Source: CAD feature listing. Evaluate the final solid. Frame: model axes, mm. A direction names the side the tool comes from. Give positions to 0.01 mm unless a question says otherwise; leave off trailing zeros. Order: outer loops, then holes, each group sorted by start corner. A loop starts at its lowest first (then second) coordinate and runs counter-clockwise, first axis right, second up.
```python
from build123d import *

# Parameters (mm, degrees)
F0_W     = 47.625
F0_H     = 19.05
F1_DEPTH = 12.7
F3_DEPTH = 7.62
F4_W     = 19.05
F4_H     = 12.7
F5_DEPTH = 7.62
F7_DEPTH = 5.08
F8_R     = 1.27


with BuildPart() as f1:
    # F0 (on Top) → F1 (new body)
    with BuildSketch(Plane.XY):
        Rectangle(F0_W, F0_H)
    extrude(amount=F1_DEPTH)

    # F2 (on face) → F3 (cut)
    with BuildSketch(Plane.XY.offset(12.7)):
        Polygon((-17.4625, -7.62), (-2.2225, -7.62), (-2.2225, 0), (-2.2225, 7.62), (-17.4625, 7.62), align=None)
    extrude(amount=-F3_DEPTH, mode=Mode.SUBTRACT)

    # F4 (on face) → F5 (join)
    with BuildSketch(Plane(origin=(-23.8125, 0, 0), x_dir=(0, -1, 0), z_dir=(-1, 0, 0))):
        with Locations((0, 6.35)):
            Rectangle(F4_W, F4_H)
    extrude(amount=F5_DEPTH)

    # F6 (on face) → F7 (join)
    with BuildSketch(Plane.XY.offset(12.7)):
        Polygon((-28.2575, 3.175), (-31.4325, 3.175), (-31.4325, -3.175), (-25.0825, -3.175), (-25.0825, 3.175), align=None)
    extrude(amount=F7_DEPTH)

    # F8
    f8_edges = [f1.edges().sort_by_distance(p)[0] for p in [
        (-31.4325, 0, 17.78),
        (-25.0825, 0, 17.78),
        (-25.0825, -3.175, 15.24),
        (-28.2575, -3.175, 17.78),
        (-28.2575, 3.175, 17.78),
        (-31.4325, -3.175, 15.24),
        (-28.2575, -3.175, 12.7),
        (-25.0825, 0, 12.7),
        (-28.2575, 3.175, 12.7),
        (-31.4325, 3.175, 15.24),
        (-25.0825, 3.175, 15.24),
        (-31.4325, -6.35, 12.7),
        (-31.4325, 6.35, 12.7),
    ]]
    fillet(f8_edges, radius=F8_R)


solid = f1.part
```
1) Section query A-A, the plane z = 6. Return the cut outline in (x, y) (1 decimal).
Report:
outline: (-31.4, -9.5) - (23.8, -9.5) - (23.8, 9.5) - (-31.4, 9.5) - close; hole (-17.5, -7.6) - (-2.2, -7.6) - (-2.2, 7.6) - (-17.5, 7.6) - close
2) Section query B-B, the plane y = -5.25. Return the cut outline in (x, z), and give its area (3 significant figures).
Report:
outline: (-31.43, 0) - (23.81, 0) - (23.81, 12.7) - (-2.22, 12.7) - (-2.22, 5.08) - (-17.46, 5.08) - (-17.46, 12.7) - (-30.16, 12.7) arc R1.27 ccw to (-31.43, 11.43) - close
area: 585 mm2
3) Reachability of faces 5 (the cylindrical face through (-31.07, -7.02, 12.32)), 6 (the flat face through (-25.082, 0, 15)), 7 (the cylindrical face through (-31.07, 2.793, 15.258)) from +Z, -Z, +X, -X, +Y, -Y: full face, straight path, thin tool, end or side. Return the list, or none.
Report:
face 5: +Z, -X, -Y
face 6: +Z, +X, +Y, -Y
face 7: +Z, -X, +Y
4) Pin query (flat end, axial travel): pin 1 (2 mm diameter, centred on y = -0.5, z = 15.5, fed in from +X); pin 2 (2 mm diameter, centred on x = -29, z = 15, fed in from +Y) (3 decimals); pin 3 (2 mm diameter, centred on x = -27.5, z = 16, fed in from -Y) (3 decimals). Return the tip coordinate at first contact, or that it passes through.
Report:
pin 1: stops at x = -25.08
pin 2: stops at y = 3.175
pin 3: stops at y = -3.175
5) Section query D-D, the plane z = 15. Return the cut outline in (x, y) (1 decimal), and give its area (3 significant figures).
Report:
outline: (-31.4, -1.9) arc R1.3 ccw to (-30.2, -3.2) - (-26.4, -3.2) arc R1.3 ccw to (-25.1, -1.9) - (-25.1, 1.9) arc R1.3 ccw to (-26.4, 3.2) - (-30.2, 3.2) arc R1.3 ccw to (-31.4, 1.9) - close
area: 38.9 mm2
6) Section query C-C, the plane x = -10. Return the cut outline in (y, z) (3 decimals).
Report:
outline: (-9.525, 0) - (9.525, 0) - (9.525, 12.7) - (7.62, 12.7) - (7.62, 5.08) - (-7.62, 5.08) - (-7.62, 12.7) - (-9.525, 12.7) - close
7) Draft query along Y for faces 1 (the flat face through (-3, 9.525, 6)), 2 (the cylindrical face through (-24.7, 0.03, 13.06)), 3 (the flat face through (-10, 7.62, 9)), 4 (the flat face through (-28, -3.175, 15)). Return one class per face: +Y half, -Y half, draft (parallel to the pull), parting line (faces both ways), or undercut.
Report:
face 1: +Y half
face 2: draft
face 3: undercut
face 4: -Y half
8) Material intervals for L1, parallel to Y at x = -8, z = 7 (3 decimals); L2, parallel to X at y = -6.25, z = 11.25; L3, parallel to Z at x = -13.5, y = 3.5, sorted ascending.
Report:
L1: y = -9.525 to -7.62, 7.62 to 9.525
L2: x = -31.43 to -17.46, -2.22 to 23.81
L3: z = 0 to 5.08
